Model file for the job. Use its own axes, mm. Round coordinates to 2 decimals unless told otherwise and drop trailing zeros. Order: outer loops, then holes, each group sorted by start corner. A loop starts at its lowest first (then second) coordinate and runs counter-clockwise, first axis right, second up. Notation, with made-up numbers: (34.25, 30.5) -> (67.25, 30.5) arc R19 cw to (67.25, 52.5) -> close; hole circle Ø5 at (30, -11). An arc over 180 degrees is marked (long way). Use CSV: the item, a comma, the result in double quotes.
Autodesk Inventor part; units mm, degrees
ref_plane "YZ Plane" through (0, 0, 0) normal (1, 0, 0) x (0, 1, 0)
ref_plane "XZ Plane" through (0, 0, 0) normal (0, 1, 0) x (-1, 0, 0)
ref_plane "XY Plane" through (0, 0, 0) normal (0, 0, 1) x (1, 0, 0)
sketch "スケッチ1" plane through (0, 0, 0) normal (0, 0, 1) x (1, 0, 0)
  circle A0 centre (-17.6777, 17.6777) radius 1.5
  circle A1 centre (17.6777, -17.6777) radius 1.5
  circle A2 centre (-17.6777, -17.6777) radius 1.5
  circle A3 centre (17.6777, 17.6777) radius 1.5
  line L0 (45, 40) -> (-45, 40)
  line L1 (-45, 40) -> (-45, -40)
  line L2 (-45, -40) -> (45, -40)
  line L3 (45, -40) -> (45, 40)
  line L4 (-5.5, 19.2289) -> (-5.5, 28)
  line L5 (-5.5, 28) -> (5.5, 28)
  line L6 (5.5, 28) -> (5.5, 19.2289)
  arc A4 (-5.5, 19.2289) -> (5.5, 19.2289) centre (0, 0) ccw
extrude "押し出し1" add sketch "スケッチ1" along normal blind 5
sketch "スケッチ2" plane through (0, 0, 0) normal (0, 0, -1) x (-1, 0, 0)
  line L0 (-5.5, 28) -> (5.5, 28)
  line L1 (5.5, 28) -> (5.5, 19.2289)
  arc A0 (-5.5, 19.2289) -> (5.5, 19.2289) centre (0, 0) ccw
  line L2 (-5.5, 19.2289) -> (-5.5, 28)
  circle A1 centre (0, 0) radius 20
  line L3 (-5.5, 19.2289) -> (-5.5, 28)
  line L4 (5.5, 28) -> (5.5, 19.2289)
extrude "押し出し2" add sketch "スケッチ2" against normal blind 5 contours L0 L1 A1 L2
sketch "スケッチ3" plane through (0, 0, 0) normal (0, 0, -1) x (-1, 0, 0)
  circle A0 centre (0, 0) radius 20
  circle A1 centre (0, 0) radius 20
extrude "押し出し3" add sketch "スケッチ3" against normal blind 5
sketch "スケッチ4" plane through (0, 0, 5) normal (0, 0, 1) x (1, 0, 0)
  line L0 (-45, -40) -> (45, -40)
  line L1 (45, -40) -> (45, 40)
  line L2 (0, -40) -> (0, -20)
  line L3 (0, -20) -> (-10, -20)
  line L4 (-10, -20) -> (10, -20)
  line L5 (-45, -40) -> (-35, -40)
  line L6 (-35, -40) -> (-35, -30)
  line L7 (-35, -30) -> (-45, -30)
  line L8 (-45, -30) -> (-45, -40)
  line L9 (45, -40) -> (35, -40)
  line L10 (35, -40) -> (35, -30)
  line L11 (35, -30) -> (45, -30)
  line L12 (45, -30) -> (45, -40)
  point P0 (0, 0)
  dimension "d6" = 20
  dimension "d7" = 10
  dimension "d8" = 20
  dimension "d9" = 10
  dimension "d10" = 10
  dimension "d11" = 10
  dimension "d12" = 10
hole "穴1" at (-35, -30, 5) at (-10, -20, 5) at (0, -20, 5) at (10, -20, 5) at (35, -30, 5) direction (0, 0, -1) diameter 3 depth 8 tip angle 118
sketch "スケッチ5" plane through (0, 0, 5) normal (0, 0, 1) x (1, 0, 0)
  circle A0 centre (0, 0) radius 7
  dimension "d20" = 14
sketch "スケッチ6" plane through (0, 0, 5) normal (0, 0, 1) x (1, 0, 0)
  circle A0 centre (10, -20) radius 1.5
  circle A1 centre (-10, -20) radius 1.5
  circle A2 centre (-35, -30) radius 1.5
  circle A3 centre (0, -20) radius 1.5
  circle A4 centre (35, -30) radius 1.5
  circle A5 centre (17.6777, 17.6777) radius 1.5
  circle A6 centre (-17.6777, -17.6777) radius 1.5
  circle A7 centre (17.6777, -17.6777) radius 1.5
  circle A8 centre (-17.6777, 17.6777) radius 1.5
  line L0 (45, 40) -> (-45, 40)
  line L1 (-45, 40) -> (-45, -40)
  line L2 (-45, -40) -> (45, -40)
  line L3 (45, -40) -> (45, 40)
  point P0 (0, 0)
extrude "押し出し4" add sketch "スケッチ5" along normal blind 80
sketch "スケッチ7" plane through (0, 0, 0) normal (0, 0, -1) x (-1, 0, 0)
  line L0 (-45, 40) -> (-35, 40)
  line L1 (-35, 40) -> (-35, 30)
  line L2 (-35, 30) -> (-45, 30)
  line L3 (-45, 30) -> (-45, 40)
  line L4 (45, 40) -> (35, 40)
  line L5 (35, 40) -> (35, 30)
  line L6 (35, 30) -> (45, 30)
  line L7 (45, 30) -> (45, 40)
  point P0 (0, 0)
  dimension "d24" = 10
  dimension "d25" = 10
  dimension "d26" = 10
  dimension "d27" = 10
hole "穴2" at (35, 30, 0) at (-35, 30, 0) direction (0, 0, 1) diameter 3 depth 8 tip angle 118
properties part number "知能ロボコンばね受け受け" material "ABS プラスチック"
Q1. Cut at D-D (y = -2). Give the cut face in (x, z), plus the area to 3 significant figures.
From the geometry:
outline,"(-45, 0) -> (45, 0) -> (45, 5) -> (6.71, 5) -> (6.71, 85) -> (-6.71, 85) -> (-6.71, 5) -> (-45, 5) -> close"
area,"1,520 mm²"
Q2. Cut at B-B (x = 35). Give the cut face in (y, z), plus the area to 3 significant figures.
From the geometry:
outline,"(-40, 0) -> (-31.5, 0) -> (-31.5, 5) -> (-40, 5) -> close; (-28.5, 0) -> (28.5, 0) -> (28.5, 5) -> (-28.5, 5) -> close; (31.5, 0) -> (40, 0) -> (40, 5) -> (31.5, 5) -> close"
area,"370 mm²"
Q3. Probe line 1 along X through (y, z) = (-20, 3.6); line 2 along Y through (x, z) = (-35, 1.4); line 3 along Z through (x, y) = (38, 31.5). List the from-to ranges inside material, lowest first.
From the geometry:
line 1,"x = -45 to -11.5, -8.5 to -1.5, 1.5 to 8.5, 11.5 to 45"
line 2,"y = -40 to -31.5, -28.5 to 28.5, 31.5 to 40"
line 3,"z = 0 to 5"
Q4. Pin check, flat tip, straight feed: pin 1 (5 mm diameter, centred on x = -35, y = -30, fed in from +Z). Stop position of the tip, or through.
From the geometry:
pin 1,"stops at z = 5"
Q5. Cut at C-C (x = 10). Give the cut face in (y, z), plus the area to 3 significant figures.
From the geometry:
outline,"(-40, 0) -> (-21.5, 0) -> (-21.5, 5) -> (-40, 5) -> close; (-18.5, 0) -> (40, 0) -> (40, 5) -> (-18.5, 5) -> close"
area,"385 mm²"
Q6. Cut at A-A (y = 30). Give the cut face in (x, z).
From the geometry:
outline,"(-45, 0) -> (-36.5, 0) -> (-36.5, 5) -> (-45, 5) -> close; (-33.5, 0) -> (33.5, 0) -> (33.5, 5) -> (-33.5, 5) -> close; (36.5, 0) -> (45, 0) -> (45, 5) -> (36.5, 5) -> close"
Q7. Mould opens along X. For faces 1 (the cylindrical face through (-18.78, 16.66, 2.46)), 2 (the cylindrical face through (6.466, 2.681, 44.44)), 3 (the flat face through (45, -1, 2)), 4 (the flat face through (1, 1, 0)) say: +X half, -X half, draft (parallel to the pull), parting line (faces both ways), or undercut.
From the geometry:
face 1,"undercut"
face 2,"parting line"
face 3,"+X half"
face 4,"draft"
